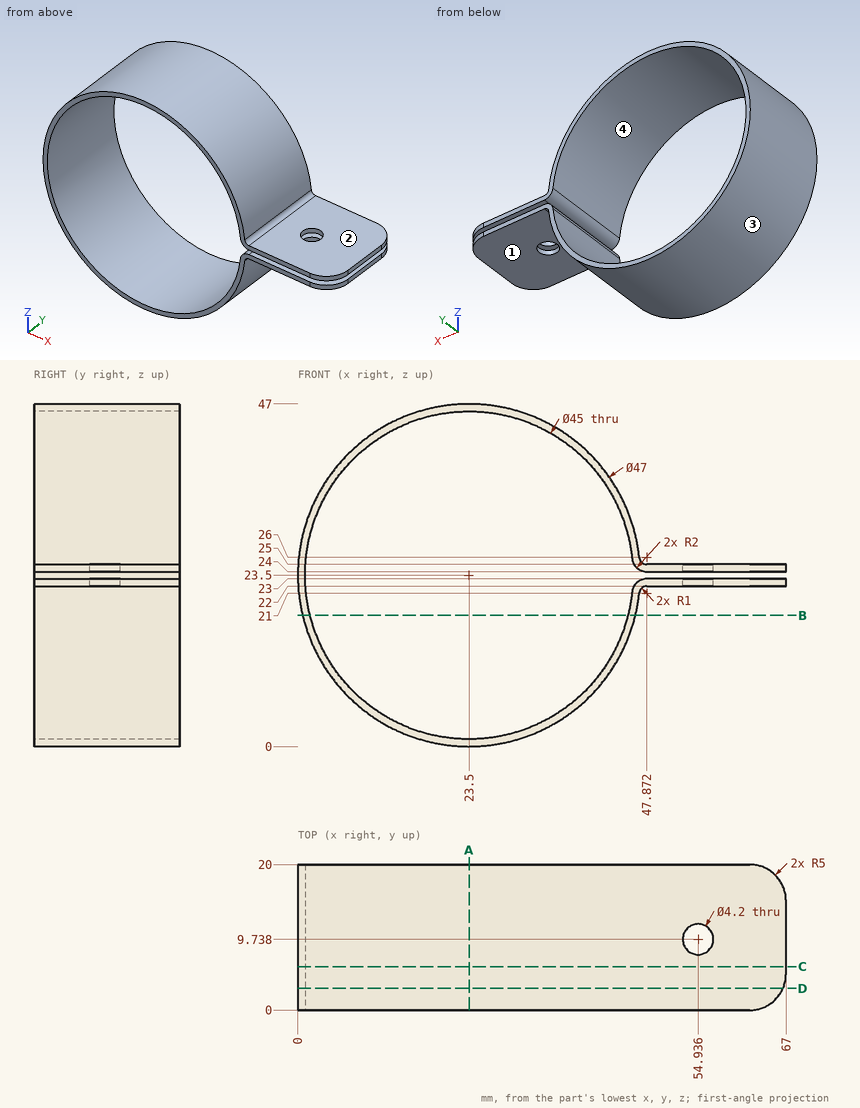
Geometry: see drawing. Coordinates: mm, zero at the bounding-box minimum. Round coordinates to 2 decimals unless told otherwise and drop trailing zeros. Loops run counter-clockwise (first coordinate to the right, second up) from the corner with the lowest first, then second, coordinate; pieces in that order, holes last. Notation, with made-up numbers: (88, 60) -> (105, 60) arc R6 cw to (105, 69) -> close; hole circle Ø7 at (70.5, 60). An arc over 180 degrees is marked (long way). Use one line per item in the form item = value. Start each with the question number.
Item 1: Material intervals for L1, parallel to Z at x = 23.5, y = 6; L2, parallel to Z at x = 49, y = 11.25; L3, parallel to X at y = 12.5, z = 23.5, sorted ascending. Write a range as from..to.
Item 2: Section query D-D on y = 3. Return the cut outline in (x, z).
Item 3: Section query C-C on y = 6. Return the cut outline in (x, z).
Item 4: Contact query for flat-ended pins moving along their axis: pin 1 Ø1.5 at (y, z) = (9, 21) entering from +X; pin 2 Ø1.5 at (y, z) = (5.5, 12) entering from -X; pin 3 Ø8 at (x, y) = (59.5, 10) entering from +Z; pin 4 Ø8 at (x, z) = (32, 36.5) entering from -Y. Output: stop coordinate, or through.
Item 5: Mould query, pull axis Z, two halves, no side actions, for the marked faces 1, 2, 3 and 4. Classes: pulls with the +Z half, pulls with the -Z half, needs draft (parallel to the pull), parting line crosses it, or undercut.
Item 6: Section query A-A on x = 23.5. Return the cut outline in (y, z), then the cut area to 3 significant figures.
Item 7: Section query B-B on z = 18. Return the cut outline in (x, y).
Ans:
q1.L1 = 0..1, 46..47
q1.L2 = 22..23, 24..25
q1.L3 = 0..1
q2.outline = (45.88, 21.2) arc R22.5 cw (long way) to (45.88, 25.8) arc R2 ccw to (47.87, 24) -> (66.58, 24) -> (66.58, 25) -> (47.87, 25) arc R1 cw to (46.88, 25.9) arc R23.5 ccw (long way) to (46.88, 21.1) arc R1 cw to (47.87, 22) -> (66.58, 22) -> (66.58, 23) -> (47.87, 23) arc R2 ccw to start
q3.outline = (45.88, 21.2) arc R22.5 cw (long way) to (45.88, 25.8) arc R2 ccw to (47.87, 24) -> (67, 24) -> (67, 25) -> (47.87, 25) arc R1 cw to (46.88, 25.9) arc R23.5 ccw (long way) to (46.88, 21.1) arc R1 cw to (47.87, 22) -> (67, 22) -> (67, 23) -> (47.87, 23) arc R2 ccw to start
q4.pin_1 = 47.21
q4.pin_2 = 2.6
q4.pin_3 = 25
q4.pin_4 = through
q5.face_1 = pulls with the -Z half
q5.face_2 = pulls with the +Z half
q5.face_3 = parting line crosses it
q5.face_4 = undercut
q6.outline = (0, 0) -> (20, 0) -> (20, 1) -> (0, 1) -> close; (0, 46) -> (20, 46) -> (20, 47) -> (0, 47) -> close
q6.area = 40.0 mm^2
q7.outline = (0.65, 0) -> (1.68, 0) -> (1.68, 20) -> (0.65, 20) -> close; (45.32, 0) -> (46.35, 0) -> (46.35, 20) -> (45.32, 20) -> close
